Design review of the part built by this model. Coordinates are the model's own, in mm. Face numbers are marked on the shaded views. A direction names the side the tool comes from. Round coordinates to 2 decimals unless told otherwise and drop trailing zeros. Write each loop counter-clockwise with the first axis right and the second up, starting at its lowest first coordinate (ties: lowest second). Pieces come first, ordered by that corner, then holes.
from build123d import *

# Parameters (mm, degrees)
F0_R      = 19.5
F1_DEPTH  = 16.5
F3_R      = 9.5
F4_DEPTH  = 12
F5_R      = 2
F6_DEPTH  = 25
F7_R      = 4.5
F8_DEPTH  = 1.5
F9_R      = 2.25
F10_DEPTH = 3
F11_R     = 0.909275
F12_DEPTH = 1
F13_R     = 19
F13_R_2   = 11
F14_DEPTH = 15
F15_R     = 3
F16_DEPTH = 9.5
F17_R     = 1.75
F18_DEPTH = 13


with BuildPart() as f1:
    # F0 (on Front) → F1 (new body)
    with BuildSketch(Plane.XZ):
        Circle(F0_R)
    extrude(amount=-F1_DEPTH)

    # F3 (on face) → F4 (cut)
    with BuildSketch(Plane.XZ):
        Circle(F3_R)
    extrude(amount=-F4_DEPTH, mode=Mode.SUBTRACT)

    # F5 (on face) → F6 (cut)
    with BuildSketch(Plane.XZ.offset(-12)):
        with Locations((0, 6.819186)):
            Circle(F5_R)
        with Locations((4.821892, 4.821892)):
            Circle(F5_R)
        with Locations((6.819186, 0)):
            Circle(F5_R)
        with Locations((4.821892, -4.821892)):
            Circle(F5_R)
        with Locations((0, -6.819186)):
            Circle(F5_R)
        with Locations((-4.821892, -4.821892)):
            Circle(F5_R)
        with Locations((-6.819186, 0)):
            Circle(F5_R)
        with Locations((-4.821892, 4.821892)):
            Circle(F5_R)
    extrude(amount=-F6_DEPTH, mode=Mode.SUBTRACT)

    # F7 (on face) → F8 (join)
    with BuildSketch(Plane.XZ.offset(-12)):
        Circle(F7_R)
    extrude(amount=F8_DEPTH)

    # F9 (on face) → F10 (join)
    with BuildSketch(Plane.XZ.offset(-10.5)):
        Circle(F9_R)
    extrude(amount=F10_DEPTH)

    # F11 (on face) → F12 (join)
    with BuildSketch(Plane.XZ.offset(-10.5)):
        with Locations((0, 3.288401)):
            Circle(F11_R)
        with Locations((2.325251, 2.325251)):
            Circle(F11_R)
        with Locations((3.288401, 0)):
            Circle(F11_R)
        with Locations((2.325251, -2.325251)):
            Circle(F11_R)
        with Locations((0, -3.288401)):
            Circle(F11_R)
        with Locations((-2.325251, -2.325251)):
            Circle(F11_R)
        with Locations((-3.288401, 0)):
            Circle(F11_R)
        with Locations((-2.325251, 2.325251)):
            Circle(F11_R)
    extrude(amount=F12_DEPTH)

    # F13 (on face) → F14 (cut)
    with BuildSketch(Plane(origin=(0, 16.5, 0), x_dir=(-1, 0, 0), z_dir=(0, 1, 0))):
        Circle(F13_R)
        Circle(F13_R_2, mode=Mode.SUBTRACT)
    extrude(amount=-F14_DEPTH, mode=Mode.SUBTRACT)

    # F15 (on face) → F16 (join)
    with BuildSketch(Plane(origin=(0, 16.5, 0), x_dir=(-1, 0, 0), z_dir=(0, 1, 0))):
        Circle(F15_R)
    extrude(amount=F16_DEPTH)

    # F17 (on face) → F18 (cut)
    with BuildSketch(Plane(origin=(0, 26, 0), x_dir=(-1, 0, 0), z_dir=(0, 1, 0))):
        Circle(F17_R)
    extrude(amount=-F18_DEPTH, mode=Mode.SUBTRACT)


solid = f1.part
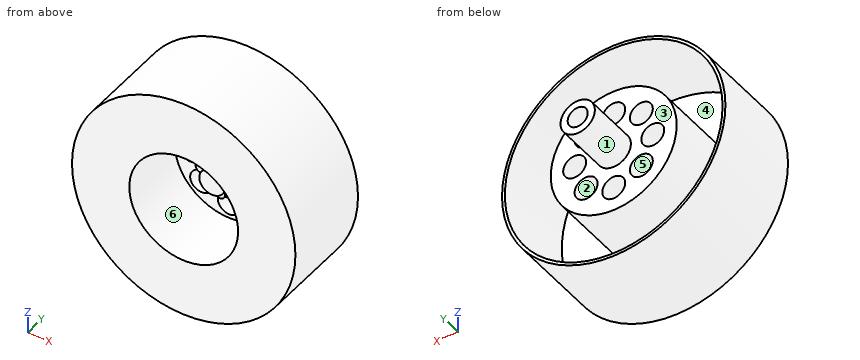
1) For P1, Ø3.5, axis at x = 4.82, z = 4.82, coming from the -Y side; P2, Ø4.5, axis at x = 4.82, z = -4.82, coming from the +Y side; P3, Ø4, axis at x = 15, z = 12, coming from the -Y side; P4, Ø1.5, axis at y = 12, z = -14, coming from the +X side, all flat-tipped, find the tip position at first contact; note any pin that passes through.
2) Add section C-C on z = 0. Count the separate pieces of the cut face and the enclosed holes in it, and give its area (3 significant figures).
3) Add section A-A on y = 11. State the section outline as (x, z) points, and give its area (3 significant figures).
4) For the marked faces 4, 5 and 6, list the 3-axis set-ups (+Z, -Z, +X, -X, +Y, -Y) from which the entire face can be reached by the end or side of a thin tool; tool diameter is ignored.
5) Add section B-B on x = -5.5. State the section outline as (y, z) points.
6) For line 1 along Z through (x, y) = (0, 13.7); line 2 along X through (y, z) = (11.25, -3); line 3 along X through (y, z) = (15, -1), list the stretches that pass through material, from the lowest coordinate up.
7) The part is to be moulded in two halves that separate along X. For the marked faces 1, 2 and 3, say which applies: pulls with the +X half, pulls with the -X half, needs draft (parallel to the pull), parting line crosses it, or undercut.
Computed:
1. P1: passes through
1. P2: stops at y = 16.5
1. P3: stops at y = 0
1. P4: stops at x = 14.31
2. separate pieces: 3
2. enclosed holes: 0
2. area: 182 mm2
3. outline: circle Ø39 at (0, 0); circle Ø22 at (0, 0); circle Ø9 at (0, 0); hole circle Ø38 at (0, 0); hole circle Ø19 at (0, 0)
3. area: 221 mm2
4. face 4: +Y
4. face 5: +Y, -Y
4. face 6: -Y
5. outline: (0, -18.71) - (16.5, -18.71) - (16.5, -18.19) - (1.5, -18.19) - (1.5, -9.53) - (16.5, -9.53) - (16.5, -6.7) - (12, -6.7) - (12, -7.75) - (0, -7.75) - close; (0, 7.75) - (12, 7.75) - (12, 6.7) - (16.5, 6.7) - (16.5, 9.53) - (1.5, 9.53) - (1.5, 18.19) - (16.5, 18.19) - (16.5, 18.71) - (0, 18.71) - close; (12, -2.94) - (16.5, -2.94) - (16.5, -1.5) - (12, -1.5) - close; (12, 1.5) - (16.5, 1.5) - (16.5, 2.94) - (12, 2.94) - close
6. line 1: z = -19.5 to -19, -11 to -8.82, -4.82 to -1.75, 1.75 to 4.82, 8.82 to 11, 19 to 19.5
6. line 2: x = -19.27 to -18.76, -10.58 to -9.01, -3.35 to 3.35, 9.01 to 10.58, 18.76 to 19.27
6. line 3: x = -19.47 to -18.97, -10.95 to -8.55, -5.09 to -1.44, 1.44 to 5.09, 8.55 to 10.95, 18.97 to 19.47
7. face 1: parting line crosses it
7. face 2: undercut
7. face 3: needs draft
